CAD build for the part. Positions are in the model's coordinates, mm. Coordinates: 2 decimals unless noted, no trailing zeros. Loops run counter-clockwise (first coordinate to the right, second up) from the corner with the lowest first, then second, coordinate; pieces in that order, holes last.
1) Saw through at B-B, the plane x = -39. Write the cut outline in (y, z), and give its area (3 significant figures).
2) Saw through at A-A, the plane z = -60. Write the cut outline in (x, y).
3) Two-plate mould, pull along X, no slides. Class faces 1 (the flat face through (-47, 2, -59)), 2 (the cylindrical face through (-35, 1, -63)): +X half, -X half, draft (parallel to the pull), parting line (faces both ways), or undercut.
4) Pin check, flat tip, straight feed: pin 1 Ø2.5 at (x, z) = (-75.17, -117.17) entering from -Y. Stop position of the tip, or through.
5) Wall check: line 1 along X through (y, z) = (1, -60); line 2 along Z through (x, y) = (-39, 0.75); line 3 along X through (y, z) = (1, -57.5). Give the ranges that are in metal, low to high.
Autodesk Inventor part; units mm, degrees
ref_plane "YZ Plane" through (0, 0, 0) normal (1, 0, 0) x (0, 1, 0)
ref_plane "XZ Plane" through (0, 0, 0) normal (0, 1, 0) x (-1, 0, 0)
ref_plane "XY Plane" through (0, 0, 0) normal (0, 0, 1) x (1, 0, 0)
sketch "Boceto1" plane through (0, 0, 0) normal (0, 1, 0) x (-1, 0, 0)
  line L0 (0, 0) -> (78, 0)
  line L1 (78, 0) -> (78, -120)
  line L2 (78, -120) -> (0, -120)
  line L3 (0, -120) -> (0, 0)
  line L4 (39, -120) -> (39, -40.9916)
  line L5 (0, -60) -> (49.8561, -60)
  circle A0 centre (39, -60) radius 5
  dimension "d0" = 120
  dimension "d1" = 78
  dimension "d11" = 10
extrude "Extrusión1" add sketch "Boceto1" along normal blind 2 contours L0 L1 L2 L4 A0 L5 L3 | L5 A0 L4 L2 L3
fillet "Empalme1" radius 2 4 edges at (0, 1, 0) (-78, 1, -120) (0, 1, -120) (-78, 1, 0)
sketch "Boceto2" plane through (0, 2, 0) normal (0, 1, 0) x (1, 0, 0)
  circle A0 centre (0, 0) radius 4
  line L0 (0, 0) -> (-8.4064, 8.4064)
  arc A1 (-2, 0) -> (0, 2) centre (-2, 2) ccw
  circle A2 centre (-2.8284, 2.8284) radius 1
  line L1 (0, 60) -> (-13.3552, 60)
  line L2 (-39, 120) -> (-39, 106.5507)
  circle A3 centre (0, 120) radius 4
  line L3 (0, 120) -> (-8.4064, 111.5936)
  arc A4 (0, 118) -> (-2, 120) centre (-2, 118) ccw
  circle A5 centre (-2.8284, 117.1716) radius 1
  circle A6 centre (-78, 120) radius 4
  line L4 (-78, 120) -> (-69.5936, 111.5936)
  arc A7 (-76, 120) -> (-78, 118) centre (-76, 118) ccw
  circle A8 centre (-75.1716, 117.1716) radius 1
  circle A9 centre (-78, 0) radius 4
  line L5 (-78, 0) -> (-69.5936, 8.4064)
  arc A10 (-78, 2) -> (-76, 0) centre (-76, 2) ccw
  circle A11 centre (-75.1716, 2.8284) radius 1
  dimension "d5" = 8
  dimension "d8" = 2
extrude "Extrusión2" cut sketch "Boceto2" against normal blind 2 contours A2 L0 A0 | A0 L0 A2 | A2 L0 A0 | A0 L0 A2 | A5 L3 A3 | A3 L3 A5 | A5 L3 A3 | A3 L3 A5 | A8 L4 A6 | A6 L4 A8 | A8 L4 A6 | A6 L4 A8 | A11 L5 A9 | A9 L5 A11 | A11 L5 A9 | A9 L5 A11
properties part number "Chasis Tapa Raspberry Pi"
Data:
1. outline: (0, -120) - (2, -120) - (2, -65) - (0, -65) - close; (0, -55) - (2, -55) - (2, 0) - (0, 0) - close
1. area: 220 mm2
2. outline: (-78, 0) - (-44, 0) - (-44, 2) - (-78, 2) - close; (-34, 0) - (0, 0) - (0, 2) - (-34, 2) - close
3. face 1: draft
3. face 2: undercut
4. pin 1: stops at y = 0
5. line 1: x = -78 to -44, -34 to 0
5. line 2: z = -120 to -65, -55 to 0
5. line 3: x = -78 to -43.33, -34.67 to 0
